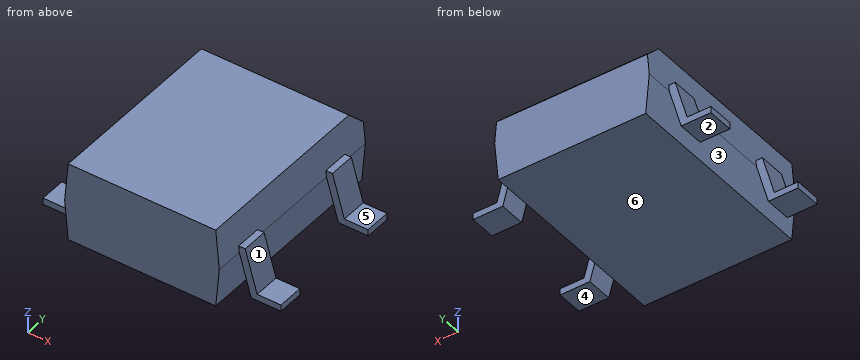
```python
from build123d import *

# Parameters (mm, degrees)
PAD001_DEPTH = 0.55
PAD002_DEPTH = 0.55
PAD_DEPTH    = 4.255
CHAMFER_SIZE = 0.75


with BuildPart() as pad001:
    # Sketch001 → Pad001 (new body, symmetric)
    with BuildSketch(Plane.XZ.offset(2.54)):
        Polygon((-5, 0), (-3.75, 0), (-3.25, 1.75), (3.25, 1.75), (3.75, 0), (5, 0), (5, 0.27), (4, 0.27), (3.5, 2.02), (-3.5, 2.02), (-4, 0.27), (-5, 0.27), align=None)
    extrude(amount=PAD001_DEPTH, both=True)


with BuildPart() as pad002:
    # Sketch002 → Pad002 (new body, symmetric)
    with BuildSketch(Plane.XZ.offset(-2.54)):
        Polygon((-5, 0), (-3.75, 0), (-3.25, 1.75), (3.25, 1.75), (3.75, 0), (5, 0), (5, 0.27), (4, 0.27), (3.5, 2.02), (-3.5, 2.02), (-4, 0.27), (-5, 0.27), align=None)
    extrude(amount=PAD002_DEPTH, both=True)


with BuildPart() as obj1:
    # Sketch → Pad (new body, symmetric)
    with BuildSketch(Plane.XZ):
        Polygon((-3.1, 0.1), (3.1, 0.1), (3.25, 1.75), (3.1, 3.4), (-3.1, 3.4), (-3.25, 1.75), align=None)
    extrude(amount=PAD_DEPTH, both=True)

    # Chamfer
    chamfer_edges = [obj1.edges().sort_by_distance(p)[0] for p in [
        (0, 4.255, 3.4),
    ]]
    chamfer(chamfer_edges, length=CHAMFER_SIZE)

    add(pad001.part)
    add(pad002.part)


solid = obj1.part
```
The model under review builds one solid part; all positions refer to its coordinate system, in mm. Face numbers are marked on the shaded views. A direction names the side the tool comes from. Give positions to 0.01 mm unless a question says otherwise; leave off trailing zeros. Write each loop counter-clockwise with the first axis right and the second up, starting at its lowest first coordinate (ties: lowest second). Pieces come first, ordered by that corner, then holes. Notation, with made-up numbers: M 60.5,85 L 118.5,85 A26 ccw 118.5,116 Z; hole C -39.75,71 d3. An arc over 180 degrees is marked long. Answer in a Markdown table with one row per item.
Item 1: Add section D-D on z = 2.25. Give the boundary of the cut face in (x, y) (3 decimals), plus the area to 3 significant figures.
Check sheet entries:
| item | result |
|---|---|
| outline | M -3.205,-4.255 L 3.205,-4.255 L 3.205,4.255 L -3.205,4.255 Z |
| area | 54.5 mm2 |
Item 2: Tool access review of the marked faces 4, 5 and 6: name each direction out of +Z, -Z, +X, -X, +Y, -Y from which nothing blocks a thin tool from reaching the whole face with its end or side.
Check sheet entries:
| item | result |
|---|---|
| face 4 | -Z, +X, -X, +Y, -Y |
| face 5 | +Z, +X, +Y, -Y |
| face 6 | -Z, +Y, -Y |
Item 3: Draft analysis for pull direction X (two halves, no side actions). For the marked faces 1, 2 and 3, state which applies: +X half, -X half, draft (parallel to the pull), parting line (faces both ways), or undercut.
Check sheet entries:
| item | result |
|---|---|
| face 1 | +X half |
| face 2 | draft |
| face 3 | undercut |
Item 4: For line 1 along Z through (x, y) = (1.75, -0.5); line 2 along X through (y, z) = (-1, 2.8); line 3 along Z through (x, y) = (0.5, 4) (3 decimals), list the stretches that pass through material, from the lowest coordinate up.
Check sheet entries:
| item | result |
|---|---|
| line 1 | 0.1 to 3.4 |
| line 2 | -3.15 to 3.15 |
| line 3 | 0.1 to 2.905 |
Item 5: Add section A-A on z = 1. Give the boundary of the cut face in (x, y) (3 decimals), plus the area to 3 significant figures.
Check sheet entries:
| item | result |
|---|---|
| outline | M -3.791,-3.09 L -3.464,-3.09 L -3.464,-1.99 L -3.791,-1.99 Z; M -3.791,1.99 L -3.464,1.99 L -3.464,3.09 L -3.791,3.09 Z; M -3.182,-4.255 L 3.182,-4.255 L 3.182,4.255 L -3.182,4.255 Z; M 3.464,-3.09 L 3.791,-3.09 L 3.791,-1.99 L 3.464,-1.99 Z; M 3.464,1.99 L 3.791,1.99 L 3.791,3.09 L 3.464,3.09 Z |
| area | 55.6 mm2 |
Item 6: Add section C-C on y = 3.25. Give the boundary of the cut face in (x, z), plus the area to 3 significant figures.
Check sheet entries:
| item | result |
|---|---|
| outline | M -3.25,1.75 L -3.1,0.1 L 3.1,0.1 L 3.25,1.75 L 3.1,3.4 L -3.1,3.4 Z |
| area | 21.0 mm2 |
Item 7: Add section B-B on x = 2. Give the boundary of the cut face in (y, z) (3 decimals), plus the area to 3 significant figures.
Check sheet entries:
| item | result |
|---|---|
| outline | M -4.255,0.1 L 4.255,0.1 L 4.255,2.65 L 3.505,3.4 L -4.255,3.4 Z |
| area | 27.8 mm2 |
Item 8: For P1, Ø0.9, axis at x = -4.5, z = 1.5, coming from the -Y side; P2, Ø0.8, axis at x = -4.5, y = 2.5, coming from the +Z side; P3, Ø1.4, axis at x = -4.5, z = 0.5, coming from the -Y side, all flat-tipped, find the tip position at first contact; note any pin that passes through.
Check sheet entries:
| item | result |
|---|---|
| P1 | through |
| P2 | z = 0.27 |
| P3 | y = -3.09 |
